from build123d import *

# Parameters (mm, degrees)
SKETCH1_R           = 3.175
BOSS_EXTRUDE1_DEPTH = 3.81
CUT_EXTRUDE1_REACH  = 334.908
SKETCH3_R           = 1.27
CUT_EXTRUDE2_REACH  = 274.112
SKETCH5_R           = 1.27
CUT_EXTRUDE3_REACH  = 334.911
SKETCH6_R           = 1.27
BOSS_EXTRUDE2_DEPTH = 3.81


with BuildPart() as part:
    # Sketch1 → Boss-Extrude1 (new body)
    with BuildSketch(Plane(origin=(0, 0, 0), x_dir=(1, 0, 0), z_dir=(0, 1, 0))):
        with BuildLine():
            Line((-132.862230357, 80.626602679), (-114.818360917, 111.876376892))
            ThreePointArc((-114.818360917, 111.876376892), (-110.170255519, 116.524341207), (-103.82099168, 118.225900714))
            Line((-103.82099168, 118.225900714), (103.762977343, 118.240259528))
            ThreePointArc((103.762977343, 118.240259528), (110.109496385, 116.541297953), (114.757781541, 111.898214981))
            Line((114.757781541, 111.898214981), (132.857908371, 80.600189632))
            ThreePointArc((132.857908371, 80.600189632), (134.563982049, 74.246129937), (132.86180691, 67.891024761))
            Line((132.86180691, 67.891024761), (29.0379736, -111.891469007))
            ThreePointArc((29.0379736, -111.891469007), (24.389544583, -116.539131318), (18.040149336, -118.240259558))
            Line((18.040149336, -118.240259558), (-18.094408415, -118.240259558))
            ThreePointArc((-18.094408415, -118.240259558), (-24.445497205, -116.538153501), (-29.09418809, -111.888081791))
            Line((-29.09418809, -111.888081791), (-132.863762321, 67.928304298))
            ThreePointArc((-132.863762321, 67.928304298), (-134.563982554, 74.277658701), (-132.862230357, 80.626602679))
        make_face()
        with Locations(Location((-103.330851621, 84.381028983, 0), (0, 0, 90))):
            Circle(SKETCH1_R, mode=Mode.SUBTRACT)
        with Locations(Location((-0.028433279, -94.702561062, 0), (0, 0, 90))):
            Circle(SKETCH1_R, mode=Mode.SUBTRACT)
        with Locations(Location((103.336854698, 84.397127461, 0), (0, 0, 90))):
            Circle(SKETCH1_R, mode=Mode.SUBTRACT)
        with BuildLine():
            Line((-84.013266269, 67.022348434), (-78.642736989, 76.323448067))
            ThreePointArc((-78.642736989, 76.323448067), (-73.995553024, 80.970880326), (-67.647495776, 82.672971564))
            Line((-67.647495776, 82.672971564), (67.773359352, 82.705030032))
            ThreePointArc((67.773359352, 82.705030032), (74.121084724, 81.006600385), (78.770291575, 76.36298581))
            Line((78.770291575, 76.36298581), (84.141622987, 67.075091406))
            ThreePointArc((84.141622987, 67.075091406), (85.847697169, 60.718674744), (84.143163353, 54.361844845))
            Line((84.143163353, 54.361844845), (16.352129804, -62.925309178))
            ThreePointArc((16.352129804, -62.925309178), (11.704017593, -67.570067982), (5.356663713, -69.27001804))
            Line((5.356663713, -69.27001804), (-5.379766134, -69.27001804))
            ThreePointArc((-5.379766134, -69.27001804), (-11.731679612, -67.567435699), (-16.380497701, -62.916190507))
            Line((-16.380497701, -62.916190507), (-84.015750126, 54.325699819))
            ThreePointArc((-84.015750126, 54.325699819), (-85.715018316, 60.674356799), (-84.013266269, 67.022348434))
        make_face(mode=Mode.SUBTRACT)
    extrude(amount=BOSS_EXTRUDE1_DEPTH)

    # Sketch3 → Cut-Extrude1 (cut, up to next)
    with BuildSketch(Plane(origin=(134.490180652, 0, -77.777728789), x_dir=(-0.5006264112230908, 0, -0.8656634429071663), z_dir=(0.8656634429071663, 0, -0.5006264112230908)), mode=Mode.PRIVATE) as cut_extrude1_sk1:
        with Locations((9.583713099, 1.905)):
            Circle(SKETCH3_R)
    cut_extrude1_tool1 = extrude(cut_extrude1_sk1.sketch, amount=-CUT_EXTRUDE1_REACH, mode=Mode.PRIVATE) & part.part
    # Sketch3 → Cut-Extrude1 (cut, up to next)
    with BuildSketch(Plane(origin=(134.490180652, 0, -77.777728789), x_dir=(-0.5006264112230908, 0, -0.8656634429071663), z_dir=(0.8656634429071663, 0, -0.5006264112230908)), mode=Mode.PRIVATE) as cut_extrude1_sk2:
        with Locations((33.073860572, 1.905)):
            Circle(SKETCH3_R)
    cut_extrude1_tool2 = extrude(cut_extrude1_sk2.sketch, amount=-CUT_EXTRUDE1_REACH, mode=Mode.PRIVATE) & part.part
    add(cut_extrude1_tool1.solids().sort_by_distance((129.692321, 1.905, -86.073999))[0], mode=Mode.SUBTRACT)
    add(cut_extrude1_tool2.solids().sort_by_distance((117.932533, 1.905, -106.408561))[0], mode=Mode.SUBTRACT)

    # Sketch5 → Cut-Extrude2 (cut, up to next)
    with BuildSketch(Plane.XY.offset(118.240259558), mode=Mode.PRIVATE) as cut_extrude2_sk1:
        with Locations((-11.784935705, 1.905)):
            Circle(SKETCH5_R)
    cut_extrude2_tool1 = extrude(cut_extrude2_sk1.sketch, amount=-CUT_EXTRUDE2_REACH, mode=Mode.PRIVATE) & part.part
    # Sketch5 → Cut-Extrude2 (cut, up to next)
    with BuildSketch(Plane.XY.offset(118.240259558), mode=Mode.PRIVATE) as cut_extrude2_sk2:
        with Locations((11.705218914, 1.905)):
            Circle(SKETCH5_R)
    cut_extrude2_tool2 = extrude(cut_extrude2_sk2.sketch, amount=-CUT_EXTRUDE2_REACH, mode=Mode.PRIVATE) & part.part
    add(cut_extrude2_tool1.solids().sort_by_distance((-11.784936, 1.905, 118.24026))[0], mode=Mode.SUBTRACT)
    add(cut_extrude2_tool2.solids().sort_by_distance((11.705219, 1.905, 118.24026))[0], mode=Mode.SUBTRACT)

    # Sketch6 → Cut-Extrude3 (cut, up to next)
    with BuildSketch(Plane(origin=(-134.555779523, 0, -77.693582727), x_dir=(-0.500037491916206, 0, 0.8660037567344326), z_dir=(-0.8660037567344328, 0, -0.500037491916206)), mode=Mode.PRIVATE) as cut_extrude3_sk1:
        with Locations((-33.174438242, 1.905)):
            Circle(SKETCH6_R)
    cut_extrude3_tool1 = extrude(cut_extrude3_sk1.sketch, amount=-CUT_EXTRUDE3_REACH, mode=Mode.PRIVATE) & part.part
    # Sketch6 → Cut-Extrude3 (cut, up to next)
    with BuildSketch(Plane(origin=(-134.555779523, 0, -77.693582727), x_dir=(-0.500037491916206, 0, 0.8660037567344326), z_dir=(-0.8660037567344328, 0, -0.500037491916206)), mode=Mode.PRIVATE) as cut_extrude3_sk2:
        with Locations((-9.684283586, 1.905)):
            Circle(SKETCH6_R)
    cut_extrude3_tool2 = extrude(cut_extrude3_sk2.sketch, amount=-CUT_EXTRUDE3_REACH, mode=Mode.PRIVATE) & part.part
    add(cut_extrude3_tool1.solids().sort_by_distance((-117.967317, 1.905, -106.422771))[0], mode=Mode.SUBTRACT)
    add(cut_extrude3_tool2.solids().sort_by_distance((-129.713275, 1.905, -86.080209))[0], mode=Mode.SUBTRACT)

    # Sketch7 → Boss-Extrude2 (add)
    with BuildSketch(Plane(origin=(0, 0, 0), x_dir=(1, 0, 0), z_dir=(0, 1, 0))):
        with BuildLine():
            Line((84.141622987, 67.075091406), (78.770291575, 76.36298581))
            ThreePointArc((78.770291575, 76.36298581), (74.121084724, 81.006600385), (67.773359352, 82.705030032))
            Line((67.773359352, 82.705030032), (-67.647495776, 82.672971564))
            ThreePointArc((-67.647495776, 82.672971564), (-73.995553024, 80.970880326), (-78.642736989, 76.323448067))
            Line((-78.642736989, 76.323448067), (-84.013266269, 67.022348434))
            ThreePointArc((-84.013266269, 67.022348434), (-85.715018316, 60.674356799), (-84.015750126, 54.325699819))
            Line((-84.015750126, 54.325699819), (-16.380497701, -62.916190507))
            ThreePointArc((-16.380497701, -62.916190507), (-11.731679612, -67.567435699), (-5.379766134, -69.27001804))
            Line((-5.379766134, -69.27001804), (5.356663713, -69.27001804))
            ThreePointArc((5.356663713, -69.27001804), (11.704017593, -67.570067982), (16.352129804, -62.925309178))
            Line((16.352129804, -62.925309178), (84.143163353, 54.361844845))
            ThreePointArc((84.143163353, 54.361844845), (85.847697169, 60.718674744), (84.141622987, 67.075091406))
        make_face()
    extrude(amount=BOSS_EXTRUDE2_DEPTH)


solid = part.part
The listing builds one solid part. Answer for the finished solid, in the listing's coordinates (mm). Round coordinates to 2 decimals unless told otherwise and drop trailing zeros. Order: outer loops, then holes, each group sorted by start corner. A loop starts at its lowest first (then second) coordinate and runs counter-clockwise, first axis right, second up. Notation, with made-up numbers: (-0.75, 59.5) -> (35.25, 59.5) arc R17 ccw to (35.25, 92.5) -> close; hole circle Ø3 at (11, 18). An arc over 180 degrees is marked (long way). Put each result on its own line as item: value.
Q1. Section D-D, the plane x = 94.5 is taken. Count the separate pieces of the cut face and the enclosed holes in it, and give its area (3 significant figures).
Results list:
separate pieces: 1
enclosed holes: 2
area: 433 mm^2
Q2. Consider line 1 along X through (y, z) = (1.55, -80); line 2 along X through (y, z) = (2.35, 102.5); line 3 along Z through (x, y) = (6.5, 3.15). Determine where each line is inside the solid, lowest interval first.
Results list:
line 1: -133.2 to -121.62, -116.74 to 116.75, 121.63 to 133.18
line 2: -34.51 to -12.97, -10.6 to 10.52, 12.89 to 34.46
line 3: -118.23 to 118.24
Q3. Section A-A, the plane z = 81 is taken. Write down the section's boundary in (x, y) (3 decimals).
Results list:
outline: (-46.919, 0) -> (46.878, 0) -> (46.878, 3.81) -> (-46.919, 3.81) -> close; hole circle Ø2.54 at (-11.785, 1.905); hole circle Ø2.54 at (11.705, 1.905)
Q4. Each of these flat-tipped pins is pushed along its axis until it touches: P1, Ø2, axis at x = 34.5, y = 2, coming from the +Z side (3 decimals); P2, Ø1.5, axis at y = 2, z = 63, coming from the -X side; P3, Ø4, axis at x = 103.34, z = -84.4, coming from the +Y side; P4, Ø7.5, axis at x = -103.33, z = -84.38, coming from the -Y side. Where does it stop, or does it pass through?
Results list:
P1: z = 104.165
P2: x = -57.74
P3: through
P4: y = 0
Q5. Determine the mould class of faces 1 (the cylindrical face through (-110.25, 1.88, -116.48)), 2 (the flat face through (2, 3.81, -28)), 3 (the cylindrical face through (101.19, 1.88, -82.06)) for opening direction Z: pulls with the +Z half, pulls with the -Z half, needs draft (parallel to the pull), parting line crosses it, or undercut.
Results list:
face 1: pulls with the -Z half
face 2: needs draft
face 3: undercut
Q6. Section B-B, the plane x = -39.5 is taken. Write down the section's boundary in (y, z), and give its area (3 significant figures).
Results list:
outline: (0, -118.23) -> (3.81, -118.23) -> (3.81, 93.86) -> (0, 93.86) -> close
area: 808 mm^2
Q7. Section C-C, the plane z = 47 is taken. Write down the section's boundary in (x, y).
Results list:
outline: (-66.54, 0) -> (66.51, 0) -> (66.51, 3.81) -> (-66.54, 3.81) -> close
